Design review of the part built by this model. Coordinates are the model's own, in mm. Give positions to 0.01 mm unless a question says otherwise; leave off trailing zeros. Order: outer loops, then holes, each group sorted by start corner. A loop starts at its lowest first (then second) coordinate and runs counter-clockwise, first axis right, second up. Notation, with made-up numbers: M -17.5,0 L 2.5,0 A23 ccw 2.5,26 Z; hole C 60,78.25 d3. An arc over 180 degrees is marked long. Answer as a JSON object with one key per item and string values.
from build123d import *

# Parameters (mm, degrees)
SKETCH1_R           = 0.762
BOSS_EXTRUDE1_DEPTH = 0.508
SKETCH2_R           = 0.635
BOSS_EXTRUDE2_DEPTH = 25.4
SKETCH3_R           = 0.762
BOSS_EXTRUDE3_DEPTH = 0.508


with BuildPart() as part:
    # Sketch1 → Boss-Extrude1 (new body)
    with BuildSketch(Plane(origin=(0, 0, 0), x_dir=(0, 0, -1), z_dir=(1, 0, 0))):
        Circle(SKETCH1_R)
    extrude(amount=BOSS_EXTRUDE1_DEPTH)

    # Sketch2 → Boss-Extrude2 (add)
    with BuildSketch(Plane(origin=(0.508, 0, 0), x_dir=(0, 0, -1), z_dir=(1, 0, 0))):
        Circle(SKETCH2_R)
    extrude(amount=BOSS_EXTRUDE2_DEPTH)

    # Sketch3 → Boss-Extrude3 (add)
    with BuildSketch(Plane(origin=(25.908, 0, 0), x_dir=(0, 0, -1), z_dir=(1, 0, 0))):
        Circle(SKETCH3_R)
    extrude(amount=BOSS_EXTRUDE3_DEPTH)


solid = part.part
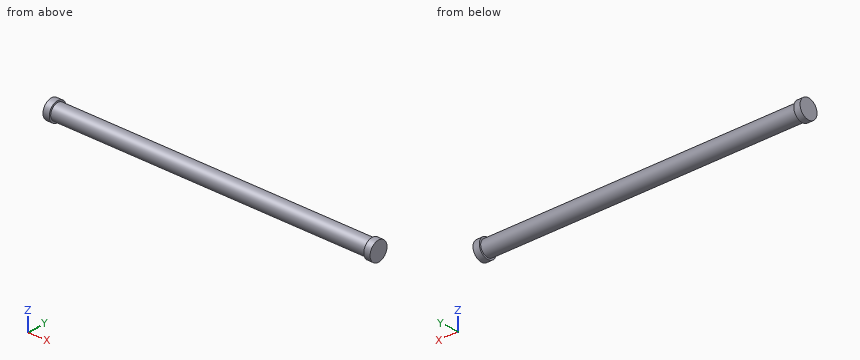
(1) We need section C-C (x = 21.75). Write out the cut boundary in (y, z) (3 decimals).
Checked values:
{"outline": "C 0,0 d1.27"}
(2) To check wall thickness, follow L1, parallel to X at y = -0.45, z = -0.55; L2, parallel to Z at x = 3.5, y = -0.05; L3, parallel to Y at x = 2.5, z = -0.4. State the ranges of each line that lie inside material, in increasing order. Write a range as from..to.
Checked values:
{"L1": "x = 0..0.51, 25.91..26.42", "L2": "z = -0.63..0.63", "L3": "y = -0.49..0.49"}
(3) We need section A-A (y = 0). Write out the cut boundary in (x, z) (3 decimals), plus the area to 3 significant figures.
Checked values:
{"outline": "M 0,-0.762 L 0.508,-0.762 L 0.508,-0.635 L 25.908,-0.635 L 25.908,-0.762 L 26.416,-0.762 L 26.416,0.762 L 25.908,0.762 L 25.908,0.635 L 0.508,0.635 L 0.508,0.762 L 0,0.762 Z", "area": "33.8 mm^2"}
